Autodesk Inventor part; units mm, degrees
ref_plane "YZ Plane" through (0, 0, 0) normal (1, 0, 0) x (0, 1, 0)
ref_plane "XZ Plane" through (0, 0, 0) normal (0, 1, 0) x (-1, 0, 0)
ref_plane "XY Plane" through (0, 0, 0) normal (0, 0, 1) x (1, 0, 0)
sketch "Sketch1" plane through (0, 0, 0) normal (0, 0, 1) x (1, 0, 0)
  circle A0 centre (0, 0) radius 5.5
  dimension "d13" = 11
extrude "Extrusion1" add sketch "Sketch1" along normal blind 25
sketch "Sketch2" plane through (0, 0, 25) normal (0, 0, 1) x (1, 0, 0)
  circle A0 centre (0, 0) radius 4
  circle A1 centre (0, 0) radius 3
  dimension "d3" = 6
extrude "Extrusion2" cut sketch "Sketch2" along normal through all both and the other way through all contours A1
sketch "Sketch3" plane through (0, 0, 0) normal (0, 1, 0) x (-1, 0, 0)
  line L0 (4, 25) -> (-4, 25)
  line L1 (0, 25) -> (0, 0)
  line L2 (0, 0) -> (0, 26.9875)
  line L3 (0, 26.9875) -> (0, -1.5875)
sketch "Sketch4" plane through (0, 0, 0) normal (1, 0, 0) x (0, 1, 0)
  point P0 (0, 0)
sketch "Sketch5" plane through (0, 0, 0) normal (0, 1, 0) x (-1, 0, 0)
  line L0 (0, 0) -> (0, 2)
  line L1 (0, 2) -> (0, 3)
  circle A0 centre (0, 3) radius 0.9
  line L2 (0, 25) -> (0, 22)
  circle A1 centre (0, 22) radius 0.9
  dimension "d6" = 2
  dimension "d7" = 1
  dimension "d8" = 1.8
  dimension "d9" = 3
  dimension "d10" = 1.8
extrude "Extrusion3" cut sketch "Sketch5" along normal through all both and the other way through all
properties part number "connector"
The listing builds one solid part. Answer for the finished solid, in the listing's coordinates (mm). Round coordinates to 2 decimals unless told otherwise and drop trailing zeros. Order: outer loops, then holes, each group sorted by start corner. A loop starts at its lowest first (then second) coordinate and runs counter-clockwise, first axis right, second up. Notation, with made-up numbers: (34.5, -26) - (83.5, -26) arc R34 ccw to (83.5, 8) - close; hole circle Ø4 at (-9, 12.5). An arc over 180 degrees is marked (long way). Write item = value, one per line. Start each with the question number.
1) Section B-B, the plane y = 0 is taken. Write down the section's boundary in (x, z).
2) Section A-A, the plane x = 0 is taken. Write down the section's boundary in (y, z), plus the area to 3 significant figures.
3) Straight lines are drawn through the part: L1, parallel to Z at x = 0, y = -4.2; L2, parallel to Y at x = 0, z = 13.75; L3, parallel to X at y = -3.65, z = 3. For each, find the intervals that lie inside material, in ascending order.
4) Given pin 1 (4 mm diameter, centred on x = -4, z = 19, fed in from +Y); pin 2 (2 mm diameter, centred on y = 3.5, z = 21.5, fed in from +X); pin 3 (6 mm diameter, centred on y = 4, z = 17.5, fed in from +X), each flat-ended and moving along its own axis, determine where each tip first touches the part or whether it passes through.
5) For a pull along X with two mould halves and no side action, classify faces 1 (the cylindrical face through (-1.19, 5.37, 12.32)), 2 (the cylindrical face through (-0.86, -4.16, 22.27)), 3 (the flat face through (2.4, -2.4, 0)) as released by +X, released by -X, zero draft, split by the parting line, or undercut.
6) Section D-D, the plane z = 5.5 is taken. Write down the section's boundary in (x, y).
7) Section C-C, the plane x = 1.75 is taken. Write down the section's boundary in (y, z), plus the area to 3 significant figures.
Results list:
q1.outline = (-5.5, 0) - (-3, 0) - (-3, 25) - (-5.5, 25) - close; (3, 0) - (5.5, 0) - (5.5, 25) - (3, 25) - close
q2.outline = (-5.5, 0) - (-3, 0) - (-3, 2.1) - (-5.5, 2.1) - close; (-5.5, 3.9) - (-3, 3.9) - (-3, 21.1) - (-5.5, 21.1) - close; (-5.5, 22.9) - (-3, 22.9) - (-3, 25) - (-5.5, 25) - close; (3, 0) - (5.5, 0) - (5.5, 2.1) - (3, 2.1) - close; (3, 3.9) - (5.5, 3.9) - (5.5, 21.1) - (3, 21.1) - close; (3, 22.9) - (5.5, 22.9) - (5.5, 25) - (3, 25) - close
q2.area = 107 mm^2
q3.L1 = 0 to 2.1, 3.9 to 21.1, 22.9 to 25
q3.L2 = -5.5 to -3, 3 to 5.5
q3.L3 = -4.11 to -0.9, 0.9 to 4.11
q4.pin_1 = 5.12
q4.pin_2 = 4.9
q4.pin_3 = 5.41
q5.face_1 = split by the parting line
q5.face_2 = undercut
q5.face_3 = zero draft
q6.outline = circle Ø11 at (0, 0); hole circle Ø6 at (0, 0)
q7.outline = (-5.21, 0) - (-2.44, 0) - (-2.44, 25) - (-5.21, 25) - close; (2.44, 0) - (5.21, 0) - (5.21, 25) - (2.44, 25) - close
q7.area = 139 mm^2
